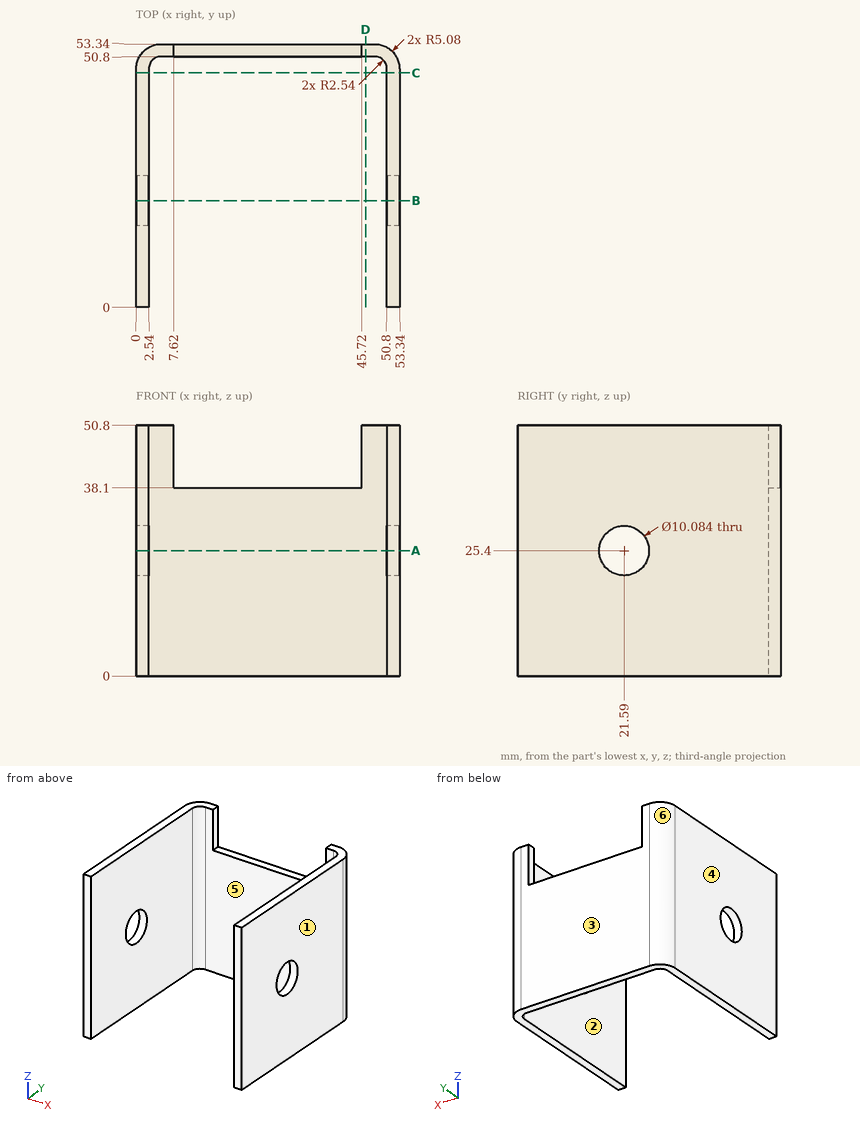
Job drawing, mm, ordinate dimensions from the low corner. One solid piece. A direction names the side the tool comes from. Give positions to 0.01 mm unless a question says otherwise; leave off trailing zeros. Write each loop counter-clockwise with the first axis right and the second up, starting at its lowest first coordinate (ties: lowest second). Pieces come first, ordered by that corner, then holes. Notation, with made-up numbers: (-17.75, -9) - (-6.75, -9) arc R21 cw to (-6.75, 28) - close; hole circle Ø4 at (14.25, 56.5). An arc over 180 degrees is marked (long way). Use one line per item in the form item = value. Start each with the question number.
1. Two-plate mould, pull along X, no slides. Class the marked faces 1, 2, 3 and 4: released by +X, released by -X, zero draft, split by the parting line, or undercut.
2. Band-saw the part on C-C on y = 47.5. Write the cut outline in (x, z), plus the area to 3 significant figures.
3. Band-saw the part on B-B on y = 21.59. Write the cut outline in (x, z).
4. Probe line 1 (X direction, y = 20, z = 46); line 2 (Y direction, x = 21, z = 12.5); line 3 (Z direction, x = 1, y = 21). List the from-to ranges inside material, lowest first. Write a range as [from, to].
5. Drop flat-ended pins along their axis: pin 1 Ø6 at (y, z) = (30, 38) entering from -X; pin 2 Ø2 at (y, z) = (51.5, 46.5) entering from +X; pin 3 Ø13 at (x, z) = (32, 30.5) entering from -Y; pin 4 Ø2 at (y, z) = (52.5, 46.5) entering from -X. Give the stop position or say it passes through.
6. Band-saw the part on A-A on z = 25.4. Write the cut outline in (x, y), plus the area to 3 significant figures.
7. Band-saw the part on D-D on x = 46.5. Write the cut outline in (y, z), plus the area to 3 significant figures.
8. 3-axis set-ups, long thin cutter, end or side, ignore diameter. For the marked faces 5 and 6: which of +Z, -Z, +X, -X, +Y, -Y reach the whole face in a straight line?
Conclusion:
q1.face_1 = released by +X
q1.face_2 = undercut
q1.face_3 = zero draft
q1.face_4 = released by -X
q2.outline = (0, 0) - (2.54, 0) - (2.54, 50.8) - (0, 50.8) - close; (50.8, 0) - (53.34, 0) - (53.34, 50.8) - (50.8, 50.8) - close
q2.area = 258 mm²
q3.outline = (0, 0) - (2.54, 0) - (2.54, 20.36) - (0, 20.36) - close; (0, 30.44) - (2.54, 30.44) - (2.54, 50.8) - (0, 50.8) - close; (50.8, 0) - (53.34, 0) - (53.34, 20.36) - (50.8, 20.36) - close; (50.8, 30.44) - (53.34, 30.44) - (53.34, 50.8) - (50.8, 50.8) - close
q4.line_1 = [0, 2.54], [50.8, 53.34]
q4.line_2 = [50.8, 53.34]
q4.line_3 = [0, 20.39], [30.41, 50.8]
q5.pin_1 = 0
q5.pin_2 = 52.82
q5.pin_3 = 50.8
q5.pin_4 = 1.17
q6.outline = (0, 0) - (2.54, 0) - (2.54, 16.55) - (0, 16.55) - close; (0, 26.63) - (2.54, 26.63) - (2.54, 48.26) arc R2.54 cw to (5.08, 50.8) - (48.26, 50.8) arc R2.54 cw to (50.8, 48.26) - (50.8, 26.63) - (53.34, 26.63) - (53.34, 48.26) arc R5.08 ccw to (48.26, 53.34) - (5.08, 53.34) arc R5.08 ccw to (0, 48.26) - close; (50.8, 0) - (53.34, 0) - (53.34, 16.55) - (50.8, 16.55) - close
q6.area = 334 mm²
q7.outline = (50.8, 0) - (53.34, 0) - (53.34, 50.8) - (50.8, 50.8) - close
q7.area = 129 mm²
q8.face_5 = +Z, -Z, -Y
q8.face_6 = +Z, -Z, -X, +Y
